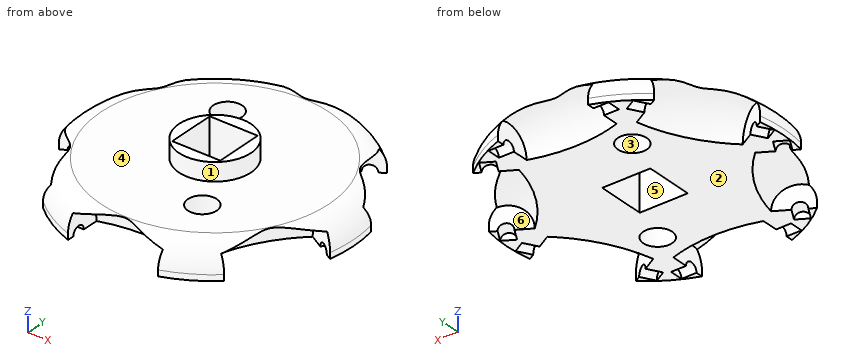
```python
from build123d import *

# Parameters (mm, degrees)
SKETCH1_R           = 18.2626
BOSS_EXTRUDE1_DEPTH = 3.96875
FILLET1_R           = 3.18516
SKETCH2_R           = 1.905
SKETCH2_W           = 6.35
SKETCH2_H           = 6.35
CUT_EXTRUDE1_DEPTH  = 27.130367418
SKETCH6_R           = 0.889
CUT_EXTRUDE2_DEPTH  = 7.9375
CIRPATTERN1_COUNT   = 6
SKETCH7_R           = 4.7625
SKETCH7_W           = 6.35
SKETCH7_H           = 6.35
BOSS_EXTRUDE2_DEPTH = 2.38125


with BuildPart() as part:
    # Sketch1 → Boss-Extrude1 (new body)
    with BuildSketch(Plane.XY):
        Circle(SKETCH1_R)
    extrude(amount=BOSS_EXTRUDE1_DEPTH)

    # Fillet1
    fillet1_edges = [part.edges().sort_by_distance(p)[0] for p in [
        (-18.2626, 0, 3.96875),
    ]]
    fillet(fillet1_edges, radius=FILLET1_R)

    # Sketch2 → Cut-Extrude1 (cut, through all)
    with BuildSketch(Plane.XY.offset(3.96875)):
        with Locations((-4.7625, 8.248891971)):
            Circle(SKETCH2_R)
        with Locations((4.7625, -8.248891971)):
            Circle(SKETCH2_R)
        Rectangle(SKETCH2_W, SKETCH2_H)
    extrude(amount=-CUT_EXTRUDE1_DEPTH, mode=Mode.SUBTRACT)

    # Sketch5 → Cut-Revolve1 (revolve, cut)
    with BuildSketch(Plane.XY):
        with BuildLine():
            Line((-5.953125, 15.46225), (5.953125, 15.46225))
            Line((5.953125, 15.46225), (5.953125, 18.496596004))
            ThreePointArc((5.953125, 18.496596004), (0, 19.431), (-5.953125, 18.496596004))
            Line((-5.953125, 18.496596004), (-5.953125, 15.46225))
        make_face()
    cut_revolve1 = revolve(axis=Axis((-5.953125, 15.46225, 0), (-1, 0, 0)), mode=Mode.SUBTRACT)

    # Sketch6 → Cut-Extrude2 (cut, symmetric)
    with BuildSketch(Plane(origin=(0, 0, 0), x_dir=(0, 0, -1), z_dir=(1, 0, 0))):
        with Locations((0, 15.46225)):
            Circle(SKETCH6_R)
    cut_extrude2 = extrude(amount=CUT_EXTRUDE2_DEPTH, both=True, mode=Mode.SUBTRACT)

    # CirPattern1: Cut-Revolve1, Cut-Extrude2 ×6 about axis
    cirpattern1_axis = Axis((0, 0, 0), (0, 0, 1))
    add([cut_revolve1.rotate(cirpattern1_axis, i * 360 / CIRPATTERN1_COUNT) for i in range(1, CIRPATTERN1_COUNT)], mode=Mode.SUBTRACT)
    add([cut_extrude2.rotate(cirpattern1_axis, i * 360 / CIRPATTERN1_COUNT) for i in range(1, CIRPATTERN1_COUNT)], mode=Mode.SUBTRACT)

    # Sketch7 → Boss-Extrude2 (add)
    with BuildSketch(Plane.XY.offset(3.96875)):
        with Locations(Location((0, 0, 0), (0, 0, 180))):
            Circle(SKETCH7_R)
        Rectangle(SKETCH7_W, SKETCH7_H, mode=Mode.SUBTRACT)
    extrude(amount=BOSS_EXTRUDE2_DEPTH)


solid = part.part
```
Here's how the part is built. I have some questions about the finished solid (model axes, mm). Face numbers are marked on the shaded views. A direction names the side the tool comes from. Coordinates: 2 decimals unless noted, no trailing zeros. Answer as CSV lines item,"result".
Q1. For the marked faces 4, 5 and 6, which set-ups out of +Z, -Z, +X, -X, +Y, -Y let a thin tool reach every point of the face, with its end or its side?
Response:
face 4,"+Z"
face 5,"+Z, -Z"
face 6,"-Z, +Y"
Q2. We'd pull the mould along X, two halves only. Please class the marked faces 1, 2 and 3: pulls with the +X half, pulls with the -X half, needs draft (parallel to the pull), parting line crosses it, or undercut.
Response:
face 1,"parting line crosses it"
face 2,"needs draft"
face 3,"undercut"
Q3. For pin 1 (8 mm diameter, centred on x = 7.5, y = 2, fed in from -Z); pin 2 (1.5 mm diameter, centred on y = 15, z = 2, fed in from +X); pin 3 (0.7 mm diameter, centred on y = -15, z = 0.5, fed in from -X); pin 4 (3 mm diameter, centred on x = 0, z = 1.5, fed in from +Y), each with a flat end and sliding along its axis, tell me the tip position at first contact or that it passes through.
Response:
pin 1,"z = 0"
pin 2,"x = 11.13"
pin 3,"x = -10.9"
pin 4,"y = 12.86"
Q4. If I drill on L1, parallel to Z at x = -14.5, y = 1; L2, parallel to X at y = -3, z = 4.75 (3 decimals); L3, parallel to X at y = 10, z = 2.75, over which ranges is the centre line in solid material (lowest first)? Write a range as [from, to].
Response:
L1,"[0, 3.97]"
L2,"[-3.699, -3.175], [3.175, 3.699]"
L3,"[-9.46, -5.51], [-4.01, 9.46]"
